from build123d import *

# Parameters (mm, degrees)
SKETCH1_W                      = 31.75
SKETCH1_H                      = 31.75
MAIN_BODY_DEPTH                = 12.7
CUT_EXTRUDE1_DEPTH             = 9.525
SKETCH3_W                      = 20
SKETCH3_H                      = 4.2545
CUT_EXTRUDE2_DEPTH             = 1.5
SKETCH4_W                      = 3.81
SKETCH4_H                      = 1.651
BOSS_EXTRUDE2_DEPTH            = 1.27
SKETCH5_R                      = 3.33375
CUT_EXTRUDE3_DEPTH             = 32.75
SKETCH6_R                      = 1.25000004
CUT_EXTRUDE4_DEPTH             = 20.32
TAP_DRILL_FOR_2_56_TAP1_D      = 1.778
TAP_DRILL_FOR_2_56_TAP2_D      = 1.778
F_3_2_3_2_DIAMETER_HOLE1_D     = 3.2
F_3_2_3_2_DIAMETER_HOLE1_DEPTH = 6.15062301
F_3_2_3_2_DIAMETER_HOLE1_TIP   = 0.96137699
TAP_DRILL_FOR_2_56_TAP4_D      = 1.778
TAP_DRILL_FOR_2_56_TAP4_DEPTH  = 6.57783491
TAP_DRILL_FOR_2_56_TAP4_TIP    = 0.53416509


with BuildPart() as part:
    # Sketch1 → Main body (new body)
    with BuildSketch(Plane(origin=(0, 0, 0), x_dir=(1, 0, 0), z_dir=(0, 1, 0))):
        with Locations((15.875, 15.875)):
            Rectangle(SKETCH1_W, SKETCH1_H)
    extrude(amount=MAIN_BODY_DEPTH)

    # Sketch2 → Cut-Extrude1 (cut)
    with BuildSketch(Plane(origin=(0, 12.7, 0), x_dir=(1, 0, 0), z_dir=(0, 1, 0))):
        Polygon((5.842, 0), (5.842, 15.24), (9.525, 15.24), (9.525, 17.712672935), (16.129, 17.712672935), (16.129, 15.24), (25.842, 15.24), (25.842, 0), align=None)
    extrude(amount=-CUT_EXTRUDE1_DEPTH, mode=Mode.SUBTRACT)

    # Sketch3 → Cut-Extrude2 (cut)
    with BuildSketch(Plane(origin=(0, 3.175, 0), x_dir=(1, 0, 0), z_dir=(0, 1, 0))):
        with Locations((15.842, 2.12725)):
            Rectangle(SKETCH3_W, SKETCH3_H)
    extrude(amount=-CUT_EXTRUDE2_DEPTH, mode=Mode.SUBTRACT)

    # Sketch4 → Boss-Extrude2 (add)
    with BuildSketch(Plane(origin=(0, 3.175, 0), x_dir=(1, 0, 0), z_dir=(0, 1, 0))):
        with Locations((12.192, 5.08)):
            Rectangle(SKETCH4_W, SKETCH4_H)
        with Locations((19.492, 5.08)):
            Rectangle(SKETCH4_W, SKETCH4_H)
    extrude(amount=BOSS_EXTRUDE2_DEPTH)

    # Sketch5 → Cut-Extrude3 (cut, through all)
    with BuildSketch(Plane.ZY):
        with Locations((-19.05, 6.35)):
            Circle(SKETCH5_R)
    extrude(amount=-CUT_EXTRUDE3_DEPTH, mode=Mode.SUBTRACT)

    # Sketch6 → Cut-Extrude4 (cut)
    with BuildSketch(Plane.ZY.offset(-31.75)):
        with Locations((-22.225, 6.35)):
            Circle(SKETCH6_R)
    extrude(amount=CUT_EXTRUDE4_DEPTH, mode=Mode.SUBTRACT)

    # Tap Drill for #2-56 Tap1 (through all)
    with Locations(Plane(origin=(0, 0, 0), x_dir=(-1, 0, 0), z_dir=(0, -1, 0))):
        with Locations((-28.575, 3.175), (-28.575, 28.575), (-3.175, 3.175), (-3.175, 28.575)):
            Hole(TAP_DRILL_FOR_2_56_TAP1_D / 2)

    # Tap Drill for #2-56 Tap2 (through all)
    with Locations(Plane(origin=(0, 3.175, 0), x_dir=(1, 0, 0), z_dir=(0, 1, 0))):
        with Locations((20.642, 8.34), (11.142, 8.34)):
            Hole(TAP_DRILL_FOR_2_56_TAP2_D / 2)

    # Ø3.2 (3.2) Diameter Hole1
    with Locations(Plane(origin=(31.75, 0, 0), x_dir=(0, 0, -1), z_dir=(1, 0, 0))):
        with Locations((28.575, 6.35), (3.175, 6.35)):
            Hole(F_3_2_3_2_DIAMETER_HOLE1_D / 2, depth=F_3_2_3_2_DIAMETER_HOLE1_DEPTH)
            with Locations((0, 0, -(F_3_2_3_2_DIAMETER_HOLE1_DEPTH + F_3_2_3_2_DIAMETER_HOLE1_TIP / 2))):  # 118° drill point
                Cone(0, F_3_2_3_2_DIAMETER_HOLE1_D / 2, F_3_2_3_2_DIAMETER_HOLE1_TIP, mode=Mode.SUBTRACT)

    # Tap Drill for #2-56 Tap4
    with Locations(Plane.ZY):
        with Locations((-3.175, 6.35), (-28.575, 6.35)):
            Hole(TAP_DRILL_FOR_2_56_TAP4_D / 2, depth=TAP_DRILL_FOR_2_56_TAP4_DEPTH)
            with Locations((0, 0, -(TAP_DRILL_FOR_2_56_TAP4_DEPTH + TAP_DRILL_FOR_2_56_TAP4_TIP / 2))):  # 118° drill point
                Cone(0, TAP_DRILL_FOR_2_56_TAP4_D / 2, TAP_DRILL_FOR_2_56_TAP4_TIP, mode=Mode.SUBTRACT)


solid = part.part
Here's how the part is built. I have some questions about the finished solid (model axes, mm). A direction names the side the tool comes from. Coordinates: 2 decimals unless noted, no trailing zeros. Loops run counter-clockwise (first coordinate to the right, second up) from the corner with the lowest first, then second, coordinate; pieces in that order, holes last. Notation, with made-up numbers: (65, 48.5) -> (87, 48.5) arc R19 ccw to (87, 63.5) -> close; hole circle Ø4 at (-26.75, 21.25). An arc over 180 degrees is marked (long way). Use one line per item in the form item = value. Start each with the question number.
(1) Will these pins go through, and if not, where does the flat tip stop? pin 1 (1.5 mm diameter, centred on x = 23.5, y = 7.5, fed in from +Z); pin 2 (1.1 mm diameter, centred on y = 6.35, z = -28.575, fed in from +X); pin 3 (1.6 mm diameter, centred on x = 3.175, z = -3.175, fed in from +Y); pin 4 (1.3 mm diameter, centred on x = 12, z = -2.5, fed in from +Y) (3 decimals).
(2) Please list where these lines run through material, in increasing order: line 1 along Y through (x, z) = (2, -19); line 2 along X through (y, z) = (10, -17) (3 decimals); line 3 along Z through (x, y) = (28, 6.75).
(3) If we section it at B-B (z = -8.34): Please give me the cut outline in (x, y) (3 decimals).
(4) On a 3-axis mill with a long thin cutter (end or side, diameter ignored), from which of +Z, -Z, +X, -X, +Y, -Y can I reach the whole of each face in a straight line? I mean faces 1 (the face through (10.287, 4, -5)), 2 (the face through (19, 4, -5.906)), 3 (the face through (11.43, 6, -23)). Say none if no direction works.
(5) If we section it at A-A (z = -19.05): Please give me the cut outline in (x, y).
(6) If we section it at C-C (y = 10.5): Please give me the cut outline in (x, z) (3 decimals).
(7) We'd pull the mould along Y, two halves only. Please class faces 4 (the face through (12, 4.445, -5)), 5 (the face through (21.732, 6.379, -23.475)), 6 (the face through (1.26, 6.62, -29.42)), 7 (the face through (13, 11, -17.713)): pulls with the +Y half, pulls with the -Y half, needs draft (parallel to the pull), parting line crosses it, or undercut.
Verdict:
q1.pin_1 = -15.24
q1.pin_2 = 24.97
q1.pin_3 = through
q1.pin_4 = 1.675
q2.line_1 = 0 to 3.02, 9.68 to 12.7
q2.line_2 = 0 to 9.525, 16.129 to 31.75
q2.line_3 = -31.75 to -30.12, -27.03 to -23.41, -15.74 to -4.72, -1.63 to 0
q3.outline = (0, 0) -> (10.253, 0) -> (10.253, 3.175) -> (5.842, 3.175) -> (5.842, 12.7) -> (0, 12.7) -> close; (12.031, 0) -> (19.753, 0) -> (19.753, 3.175) -> (12.031, 3.175) -> close; (21.531, 0) -> (31.75, 0) -> (31.75, 12.7) -> (25.842, 12.7) -> (25.842, 3.175) -> (21.531, 3.175) -> close
q4.face_1 = +Z, +Y
q4.face_2 = +Y
q4.face_3 = +Z, +X
q5.outline = (0, 0) -> (31.75, 0) -> (31.75, 3.02) -> (0, 3.02) -> close; (0, 9.68) -> (31.75, 9.68) -> (31.75, 12.7) -> (0, 12.7) -> close
q6.outline = (0, -31.75) -> (31.75, -31.75) -> (31.75, 0) -> (25.842, 0) -> (25.842, -15.24) -> (16.129, -15.24) -> (16.129, -17.713) -> (9.525, -17.713) -> (9.525, -15.24) -> (5.842, -15.24) -> (5.842, 0) -> (0, 0) -> close; hole circle Ø1.778 at (3.175, -28.575); hole circle Ø1.778 at (3.175, -3.175); hole circle Ø1.778 at (28.575, -28.575); hole circle Ø1.778 at (28.575, -3.175)
q7.face_4 = pulls with the +Y half
q7.face_5 = undercut
q7.face_6 = undercut
q7.face_7 = needs draft
